from build123d import *

# Parameters (mm, degrees)
SKETCH1_W               = 103
SKETCH1_H               = 10
CUT_EXTRUDE1_START      = -7
CUT_EXTRUDE1_DEPTH      = 14
CUT_EXTRUDE2_START      = -7
CUT_EXTRUDE2_DEPTH      = 14
CUT_EXTRUDE3_DEPTH      = 104.966340707
CUT_EXTRUDE3_DEPTH_BACK = 104.966340707
SKETCH4_R               = 5.983
CHAMFER1_SIZE           = 2


with BuildPart() as part:
    # Sketch1 → Revolve1 (revolve)
    with BuildSketch(Plane.XY, mode=Mode.PRIVATE) as revolve1_sk:
        with Locations((-51.5, 5)):
            Rectangle(SKETCH1_W, SKETCH1_H)
    revolve(revolve1_sk.sketch.rotate(Axis((-103, 0, 0), (1, 0, 0)), 90), axis=Axis((-103, 0, 0), (1, 0, 0)))

    # Sketch2 → Cut-Extrude1 (cut)
    with BuildSketch(Plane(origin=(0, 0, 0), x_dir=(0, 0, -1), z_dir=(1, 0, 0)).offset(CUT_EXTRUDE1_START)):
        with BuildLine():
            Line((-10.872335562, 5), (10.872335562, 5))
            ThreePointArc((10.872335562, 5), (0, 11.966941154), (-10.872335562, 5))
        make_face()
    extrude(amount=-CUT_EXTRUDE1_DEPTH, mode=Mode.SUBTRACT)

    # Sketch3 → Cut-Extrude2 (cut)
    with BuildSketch(Plane.ZY.offset(103).offset(CUT_EXTRUDE2_START)):
        with BuildLine():
            Line((-15, 5), (15, 5))
            ThreePointArc((15, 5), (0, 15.811388301), (-15, 5))
        make_face()
    extrude(amount=-CUT_EXTRUDE2_DEPTH, mode=Mode.SUBTRACT)

    # Sketch4 → Cut-Extrude3 (cut, two sides: drawn at the far end of the back side and taken through both)
    with BuildSketch(Plane(origin=(0, 0, 0), x_dir=(1, 0, 0), z_dir=(0, 1, 0)).offset(-CUT_EXTRUDE3_DEPTH_BACK)):
        with Locations(Location((-89, 0, 0), (0, 0, 270))):
            Circle(SKETCH4_R)
        with Locations(Location((-14, 0, 0), (0, 0, 270))):
            Circle(SKETCH4_R)
    extrude(amount=CUT_EXTRUDE3_DEPTH + CUT_EXTRUDE3_DEPTH_BACK, mode=Mode.SUBTRACT)

    # Chamfer1
    chamfer1_edges = [part.edges().sort_by_distance(p)[0] for p in [
        (0, 0, -10),
        (-103, 0, -10),
    ]]
    chamfer(chamfer1_edges, length=CHAMFER1_SIZE)


solid = part.part
Geometry: final body of the model. Coordinates: model frame, mm. A direction names the side the tool comes from. Coordinates: 2 decimals unless noted, no trailing zeros. Order: outer loops, then holes, each group sorted by start corner. A loop starts at its lowest first (then second) coordinate and runs counter-clockwise, first axis right, second up.
(1) Section query A-A (y = 0). Return the cut outline in (x, z), plus the area to 3 significant figures.
(2) Material intervals for probe 1 along X at (y, z) = (-2.5, 0); probe 2 along X at (y, z) = (7.5, -0.5); probe 3 along Z at (x, y) = (-14, -6), sorted ascending.
(3) First-contact query: pin 1 (1.5 mm diameter, centred on x = -64, z = 3.5, fed in from +Y); pin 2 (2 mm diameter, centred on x = -78, y = 7, fed in from -Z); pin 3 (8 mm diameter, centred on x = -59.5, y = -4.5, fed in from +Z). Flat tips, straight axial feed; report the tip coordinate or a pass-through.
(4) Section query D-D (x = -13). Return the cut outline in (y, z).
(5) Section query B-B (z = 0). Return the cut outline in (x, y).
(6) Access query for faces 1 (the face through (-91, 5, -6)), 2 (the face through (-50.81, -8.43, 5.38)). Directions: +Z, -Z, +X, -X, +Y, -Y. A direction counts if a zero-diameter tool reaches every point of the face in a straight line with its end or side. Return the directions, or none.
(7) Section query C-C (x = -85.5). Return the cut outline in (y, z), plus the area to 3 significant figures.
(8) Draft query along X for faces 3 (the face through (-96, 7, 0)), 4 (the face through (0, 0, 0)), 5 (the face through (-102.875, -2.441, 7.75)), 6 (the face through (-91.292, -2.613, 5.527)). Return one class per face: pulls with the +X half, pulls with the -X half, needs draft (parallel to the pull), parting line crosses it, or undercut.
Solution:
1. outline: (-103, -8) - (-101, -10) - (-2, -10) - (0, -8) - (0, 8) - (-2, 10) - (-101, 10) - (-103, 8) - close; hole circle Ø11.97 at (-89, 0); hole circle Ø11.97 at (-14, 0)
1. area: 1,830 mm2
2. probe 1: x = -103 to -94.98, -83.02 to -19.98, -8.02 to 0
2. probe 2: x = -103 to -96, -82 to -21, -7 to 0
2. probe 3: z = -8 to -5.98, 5.98 to 8
3. pin 1: stops at y = 9.61
3. pin 2: stops at z = -8
3. pin 3: stops at z = 9.99
4. outline: (-8.07, -5.9) arc R10 ccw to (5, -8.66) - (5, -5.9) - close; (-8.07, 5.9) - (5, 5.9) - (5, 8.66) arc R10 ccw to start
5. outline: (-103, -8) - (-101, -10) - (-94.98, -10) - (-94.98, 5) - (-96, 5) - (-96, 10) - (-101, 10) - (-103, 8) - close; (-83.02, -10) - (-19.98, -10) - (-19.98, 5) - (-21, 5) - (-21, 10) - (-82, 10) - (-82, 5) - (-83.02, 5) - close; (-8.02, -10) - (-2, -10) - (0, -8) - (0, 8) - (-2, 10) - (-7, 10) - (-7, 5) - (-8.02, 5) - close
6. face 1: +Z, -Z, +Y
6. face 2: +X, -X
7. outline: (-8.74, -4.85) arc R10 ccw to (5, -8.66) - (5, -4.85) - close; (-8.74, 4.85) - (5, 4.85) - (5, 8.66) arc R10 ccw to start
7. area: 111 mm2
8. face 3: undercut
8. face 4: pulls with the +X half
8. face 5: pulls with the -X half
8. face 6: undercut
